For this review, take the finished solid that the model builds, in its own axes (mm). Face numbers are marked on the shaded views. A direction names the side the tool comes from. Give positions to 0.01 mm unless a question says otherwise; leave off trailing zeros. Loops run counter-clockwise (first coordinate to the right, second up) from the corner with the lowest first, then second, coordinate; pieces in that order, holes last.
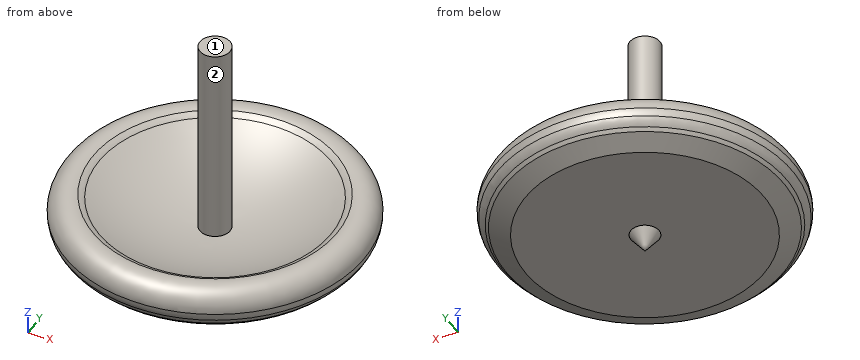
```python
from build123d import *


# Not quite as in the source:
# - a fillet or chamfer that OpenCascade refuses, or shapes differently, is made with other operations: its cross-section is extruded or revolved along the edge and cut away or added


with BuildPart() as f1:
    # F0 (on Front) → F1 (revolve)
    with BuildSketch(Plane.XZ):
        with BuildLine():
            ThreePointArc((72.7515336349, 31.5465186996), (42.1923391821, 18.1752933834), (9.525, 11.43))
            Line((9.525, 11.43), (9.525, 138.43))
            Line((9.525, 138.43), (0, 138.43))
            Line((0, 138.43), (0, 5.08))
            Line((0, 5.08), (8.89, 5.08))
            Line((8.89, 5.08), (80.9900359946, 5.08))
            ThreePointArc((80.9900359946, 5.08), (85.3313804759, 8.3219837991), (89.1588856559, 12.1570763605))
            ThreePointArc((89.1588856559, 12.1570763605), (71.2952522719, 13.6775386544), (72.7515336349, 31.5465186996))
        make_face()
        with BuildLine():
            ThreePointArc((76.5693657258, 33.7870508297), (74.5620768343, 32.8344105725), (72.7515336349, 31.5465186996))
            ThreePointArc((72.7515336349, 31.5465186996), (74.6681976781, 32.6535822964), (76.5693657258, 33.7870508297))
        make_face()
        with BuildLine():
            ThreePointArc((76.5693657258, 33.7870508297), (74.6681976781, 32.6535822964), (72.7515336349, 31.5465186996))
            ThreePointArc((72.7515336349, 31.5465186996), (71.2952522719, 13.6775386544), (89.1588856559, 12.1570763605))
            ThreePointArc((89.1588856559, 12.1570763605), (91.0491403746, 14.536624633), (92.7400229866, 17.0617442093))
            ThreePointArc((92.7400229866, 17.0617442093), (93.4502694354, 19.4251359639), (93.6900359946, 21.8812675974))
            ThreePointArc((93.6900359946, 21.8812675974), (88.2408113871, 32.3079763881), (76.5693657258, 33.7870508297))
        make_face()
        with BuildLine():
            ThreePointArc((92.7400229866, 17.0617442093), (91.0491403746, 14.536624633), (89.1588856559, 12.1570763605))
            ThreePointArc((89.1588856559, 12.1570763605), (91.2469339214, 14.3922059126), (92.7400229866, 17.0617442093))
        make_face()
        Polygon((8.89, 5.08), (0, 5.08), (0, 0), (0, -6.35), align=None)
    revolve(axis=Axis((0, 0, 4.7224786045), (0, 0, 1)))

    # F2: chamfer of 5.08 on 1 edges, made by hand

    # F2_s1 → F2_t2 (revolve, cut)
    with BuildSketch(Plane.XZ):
        with BuildLine():
            Line((74.8406610891, 5.0020764693), (87.521834843, 10.2676383795))
            Line((87.521834843, 10.2676383795), (87.5938009931, 10.1959206464))
            ThreePointArc((87.5938009931, 10.1959206464), (84.4417917383, 7.4442968535), (81.044772889, 4.9944054185))
            Line((81.044772889, 4.9944054185), (80.9900359946, 4.9784))
            ThreePointArc((80.9900359946, 4.9784), (77.9153485418, 4.9784), (74.8406610891, 4.9004764693))
            Line((74.8406610891, 4.9004764693), (74.8406610891, 5.0020764693))
        make_face()
    revolve(axis=Axis((0, 0, 5.08), (0, 0, 1)), mode=Mode.SUBTRACT)


solid = f1.part
```
Q1. For pin 1 Ø2 at (x, y) = (11.5, -22.5) entering from +Z; pin 2 Ø2 at (x, z) = (21, 26.5) entering from +Y; pin 3 Ø12 at (x, y) = (41, 17.5) entering from +Z, all flat-tipped, find the tip position at first contact; note any pin that passes through.
Answers:
pin 1: stops at z = 14
pin 2: stops at y = 90.84
pin 3: stops at z = 21.1
Q2. For probe 1 along Z at (x, y) = (-58.5, 32.5); probe 2 along Z at (x, y) = (-25.5, -66.5); probe 3 along X at (y, z) = (7, 98), list the stretches that pass through material, from the lowest coordinate up.
Answers:
probe 1: z = 5.08 to 28.39
probe 2: z = 5.08 to 30.69
probe 3: x = -6.46 to 6.46
Q3. Consider section A-A on z = 79.5. Give the boundary of the cut face in (x, y) (3 decimals).
Answers:
outline: circle Ø19.05 at (0, 0)
Q4. Machinability: for the marked faces 1 and 2, which of the approach directions +Z, -Z, +X, -X, +Y, -Y give a long, thin tool a straight path to every point of the face, cutting with its end or side? Answer none if there is none.
Answers:
face 1: +Z, +X, -X, +Y, -Y
face 2: +Z
